from build123d import *

# Parameters (mm, degrees)
SKETCH1_R           = 2.7499945
SKETCH1_R_2         = 2.75
BOSS_EXTRUDE1_DEPTH = 7
SKETCH3_R           = 7
SKETCH3_R_2         = 3.175
BOSS_EXTRUDE2_DEPTH = 8.449
SKETCH6_R           = 6.35
SKETCH6_R_2         = 3.175
BOSS_EXTRUDE4_DEPTH = 5
BOSS_EXTRUDE5_DEPTH = 10


with BuildPart() as part:
    # Sketch1 → Boss-Extrude1 (new body)
    with BuildSketch(Plane(origin=(0, 0, 0), x_dir=(0, 0, -1), z_dir=(1, 0, 0))):
        with BuildLine():
            Line((-11, 125), (11, 125))
            ThreePointArc((11, 125), (14.535533906, 123.535533906), (16, 120))
            Line((16, 120), (16, 0))
            ThreePointArc((16, 0), (0, -16), (-16, 0))
            Line((-16, 0), (-16, 120))
            ThreePointArc((-16, 120), (-14.535533906, 123.535533906), (-11, 125))
        make_face()
        with Locations((0, 107.5)):
            Circle(SKETCH1_R, mode=Mode.SUBTRACT)
        with Locations((0, 72.5)):
            Circle(SKETCH1_R_2, mode=Mode.SUBTRACT)
        with Locations((0, 12)):
            Circle(SKETCH1_R_2, mode=Mode.SUBTRACT)
        with Locations((8.485281374, 8.485281374)):
            Circle(SKETCH1_R_2, mode=Mode.SUBTRACT)
        with Locations((12, 0)):
            Circle(SKETCH1_R_2, mode=Mode.SUBTRACT)
        with Locations((8.485281374, -8.485281374)):
            Circle(SKETCH1_R_2, mode=Mode.SUBTRACT)
        with Locations((0, -12)):
            Circle(SKETCH1_R_2, mode=Mode.SUBTRACT)
        with Locations((-8.485281374, -8.485281374)):
            Circle(SKETCH1_R_2, mode=Mode.SUBTRACT)
        with Locations((-12, 0)):
            Circle(SKETCH1_R_2, mode=Mode.SUBTRACT)
        with Locations((-8.485281374, 8.485281374)):
            Circle(SKETCH1_R_2, mode=Mode.SUBTRACT)
    extrude(amount=BOSS_EXTRUDE1_DEPTH)

    # Sketch3 → Boss-Extrude2 (add)
    with BuildSketch(Plane(origin=(7, 0, 0), x_dir=(0, 0, -1), z_dir=(1, 0, 0))):
        Circle(SKETCH3_R)
        Circle(SKETCH3_R_2, mode=Mode.SUBTRACT)
    extrude(amount=BOSS_EXTRUDE2_DEPTH)

    # Sketch6 → Boss-Extrude4 (add)
    with BuildSketch(Plane(origin=(15.449, 0, 0), x_dir=(0, 0, -1), z_dir=(1, 0, 0))):
        Circle(SKETCH6_R)
        Circle(SKETCH6_R_2, mode=Mode.SUBTRACT)
    extrude(amount=BOSS_EXTRUDE4_DEPTH)

    # Sketch7 → Boss-Extrude5 (add)
    with BuildSketch(Plane(origin=(7, 0, 0), x_dir=(0, 0, -1), z_dir=(1, 0, 0))):
        with BuildLine():
            Line((-12.825, 93.175), (12.825, 93.175))
            ThreePointArc((12.825, 93.175), (16, 90), (12.825, 86.825))
            Line((12.825, 86.825), (-12.825, 86.825))
            ThreePointArc((-12.825, 86.825), (-16, 90), (-12.825, 93.175))
        make_face()
    extrude(amount=BOSS_EXTRUDE5_DEPTH)


solid = part.part
Could you check a few things on this model? Use its own coordinates, in mm. A direction names the side the tool comes from. Coordinates: 2 decimals unless noted, no trailing zeros. Order: outer loops, then holes, each group sorted by start corner. A loop starts at its lowest first (then second) coordinate and runs counter-clockwise, first axis right, second up.
Q1. Suppose I cut it at C-C on x = 5. Give the number of separate pieces and of enclosed holes in the cut face, and give its area (3 significant figures).
Q2. Please list where these lines run through material, in increasing order: L1, parallel to Y at x = 16.75, z = 0 (3 decimals); L2, parallel to Y at x = 3.25, z = 0; L3, parallel to Y at x = 4.25, z = -11.
Q3. Will these pins go through, and if not, where does the flat tip stop? pin 1 (5 mm diameter, centred on y = 91.5, z = -0.5, fed in from +X); pin 2 (6.5 mm diameter, centred on y = 0, z = 12, fed in from +X); pin 3 (3 mm diameter, centred on x = 10.5, z = -6, fed in from +Y) (3 decimals).
Q4. Suppose I cut it at B-B on y = 72.5. Please give me the cut outline in (x, z), and give its area (4 significant figures).
Q5. Which directions (+Z, -Z, +X, -X, +Y, -Y) give clear straight access to the entire face, cutting with the end or side of a thin tool? Please do faces 1 (the flat face through (7, 0, 0)), 2 (the flat face through (17, 90, 0)), 3 (the cylindrical face through (3.451, -9.539, -11.026)).
Q6. Suppose I cut it at A-A on x = 14.25. Please give me the cut outline in (y, z) (3 decimals), and give its area (3 significant figures).
Q7. Thinking about a two-plate mould opening in Z: for faces 4 (the flat face through (7, 50, 0)), 5 (the cylindrical face through (3.451, 8.606, 11.233)), 6 (the cylindrical face through (12, 90, 16)), which applies, released by +Z, released by -Z, zero draft, split by the parting line, or undercut?
Answer:
1. separate pieces: 1
1. enclosed holes: 10
1. area: 4,150 mm2
2. L1: y = -6.35 to -3.175, 3.175 to 6.35, 86.825 to 93.175
2. L2: y = -16 to -14.75, -9.25 to 9.25, 14.75 to 69.75, 75.25 to 104.75, 110.25 to 125
2. L3: y = -11.62 to -9.6, -7.37 to -2.56, 2.56 to 7.37, 9.6 to 125
3. pin 1: stops at x = 17
3. pin 2: stops at x = 7
3. pin 3: stops at y = 93.175
4. outline: (0, -16) - (7, -16) - (7, -2.75) - (0, -2.75) - close; (0, 2.75) - (7, 2.75) - (7, 16) - (0, 16) - close
4. area: 185.5 mm2
5. face 1: +X
5. face 2: +Z, -Z, +X, +Y
5. face 3: +X, -X
6. outline: circle Ø14 at (0, 0); (86.825, -12.825) arc R3.175 ccw to (93.175, -12.825) - (93.175, 12.825) arc R3.175 ccw to (86.825, 12.825) - close; hole circle Ø6.35 at (0, 0)
6. area: 317 mm2
7. face 4: zero draft
7. face 5: undercut
7. face 6: released by +Z
